Input: part model. Units: mm. Frame: model coordinates. A direction names the side the tool comes from. Coordinates: 2 decimals unless noted, no trailing zeros. Write each loop counter-clockwise with the first axis right and the second up, starting at its lowest first coordinate (ties: lowest second). Pieces come first, ordered by that corner, then holes. Notation, with made-up numbers: M 82.5,76 L 86.5,76 A22 ccw 86.5,93 Z; hole C 55,6 d9. An arc over 180 degrees is marked long. Use CSV: the item, a comma, the result in double quotes.
```python
from build123d import *

# Parameters (mm, degrees)
BOSS_EXTRUDE1_DEPTH     = 12
SKETCH5_R               = 2
CUT_EXTRUDE4_DEPTH      = 12.5
CUT_EXTRUDE6_DEPTH      = 10
CUT_EXTRUDE6_DEPTH_BACK = 16
SKETCH9_W               = 19.938266946
SKETCH9_H               = 5.5
CUT_EXTRUDE8_DEPTH      = 43.720018727
CUT_EXTRUDE8_DEPTH_BACK = 43.720018727
SKETCH7_R               = 3.15


with BuildPart() as part:
    # Sketch1 → Boss-Extrude1 (new body)
    with BuildSketch(Plane.XY):
        with BuildLine():
            Line((4.5, 40), (-4.5, 40))
            Line((-4.5, 40), (-8.942125974, 1.019010828))
            ThreePointArc((-8.942125974, 1.019010828), (0, -9), (8.942125974, 1.019010828))
            Line((8.942125974, 1.019010828), (4.5, 40))
        make_face()
    extrude(amount=BOSS_EXTRUDE1_DEPTH)

    # Sketch5 → Cut-Extrude4 (cut)
    with BuildSketch(Plane(origin=(0, 40, 0), x_dir=(1, 0, 0), z_dir=(0, 1, 0))):
        with Locations(Location((0, -6, 0), (0, 0, 270))):
            Circle(SKETCH5_R)
    extrude(amount=-CUT_EXTRUDE4_DEPTH, mode=Mode.SUBTRACT)

    # Sketch9 → Cut-Extrude6 (cut, two sides: drawn at the far end of the back side and taken through both)
    with BuildSketch(Plane(origin=(0, 0, 0), x_dir=(1, 0, 0), z_dir=(0, 1, 0)).offset(-CUT_EXTRUDE6_DEPTH_BACK)):
        with Locations((0, -6)):
            Rectangle(SKETCH9_W, SKETCH9_H)
    extrude(amount=CUT_EXTRUDE6_DEPTH + CUT_EXTRUDE6_DEPTH_BACK, mode=Mode.SUBTRACT)

    # Sketch7 → Cut-Extrude8 (cut, two sides: drawn at the far end of the back side and taken through both)
    with BuildSketch(Plane.XY.offset(-CUT_EXTRUDE8_DEPTH_BACK)):
        Circle(SKETCH7_R)
    extrude(amount=CUT_EXTRUDE8_DEPTH + CUT_EXTRUDE8_DEPTH_BACK, mode=Mode.SUBTRACT)


solid = part.part
```
1. Section A-A (y = 0). Return loops of the section in (x, z).
Resolved:
outline,"M -9,0 L -3.15,0 L -3.15,3.25 L -9,3.25 Z; M -9,8.75 L -3.15,8.75 L -3.15,12 L -9,12 Z; M 3.15,0 L 9,0 L 9,3.25 L 3.15,3.25 Z; M 3.15,8.75 L 9,8.75 L 9,12 L 3.15,12 Z"
2. Access query for faces 1 (the flat face through (6.75, 20.24, 5.92)), 2 (the flat face through (0, 5, 8.75)), 3 (the flat face through (0, 27.5, 6)). Directions: +Z, -Z, +X, -X, +Y, -Y. A direction counts if a zero-diameter tool reaches every point of the face in a straight line with its end or side. Return the directions, or none.
Resolved:
face 1,"+Z, -Z, +X, +Y"
face 2,"+X, -X, -Y"
face 3,"+Y"
3. Mould query, pull axis Z, two halves, no side actions, for faces 4 (the flat face through (0, 10, 6)), 5 (the flat face through (0, 16, 12)), 6 (the cylindrical face through (-2.5, -1.917, 1.602)). Classes: pulls with the +Z half, pulls with the -Z half, needs draft (parallel to the pull), parting line crosses it, or undercut.
Resolved:
face 4,"undercut"
face 5,"pulls with the +Z half"
face 6,"needs draft"
4. Section D-D (x = 5.25). Return loops of the section in (y, z).
Resolved:
outline,"M -7.31,0 L 33.42,0 L 33.42,12 L -7.31,12 L -7.31,8.75 L 10,8.75 L 10,3.25 L -7.31,3.25 Z"
5. Section B-B (x = 0). Return loops of the section in (y, z).
Resolved:
outline,"M -9,0 L -3.15,0 L -3.15,3.25 L -9,3.25 Z; M -9,8.75 L -3.15,8.75 L -3.15,12 L -9,12 Z; M 3.15,0 L 40,0 L 40,4 L 27.5,4 L 27.5,8 L 40,8 L 40,12 L 3.15,12 L 3.15,8.75 L 10,8.75 L 10,3.25 L 3.15,3.25 Z"
6. Section C-C (z = 6). Return loops of the section in (x, y), then the cut area to 3 significant figures.
Resolved:
outline,"M -7.92,10 L 7.92,10 L 4.5,40 L 2,40 L 2,27.5 L -2,27.5 L -2,40 L -4.5,40 Z"
area,"323 mm^2"
7. Contact query for flat-ended pins moving along their axis: pin 1 Ø2 at (y, z) = (24, 10.5) entering from +X; pin 2 Ø1.6 at (x, z) = (1.5, 5) entering from -Y; pin 3 Ø1.5 at (x, z) = (-7, 3) entering from -Y. Output: stop coordinate, or through.
Resolved:
pin 1,"stops at x = 6.44"
pin 2,"stops at y = 10"
pin 3,"stops at y = -6.48"
8. Material intervals for line 1 (Y direction, x = 0, z = 10.8); line 2 (Z direction, x = -7, y = -2); line 3 (X direction, y = 0, z = 10.3), sorted ascending. Write a range as [from, to].
Resolved:
line 1,"y = [-9, -3.15], [3.15, 40]"
line 2,"z = [0, 3.25], [8.75, 12]"
line 3,"x = [-9, -3.15], [3.15, 9]"
